CAD build for the part. Positions are in the model's coordinates, mm. Face numbers are marked on the shaded views. A direction names the side the tool comes from. Round coordinates to 2 decimals unless told otherwise and drop trailing zeros. Loops run counter-clockwise (first coordinate to the right, second up) from the corner with the lowest first, then second, coordinate; pieces in that order, holes last. Notation, with made-up numbers: M 19.25,4.5 L 49.25,4.5 A32 cw 49.25,41.5 Z; hole C 87,40 d1. An arc over 180 degrees is marked long. Put each result on its own line as item: value. Start each with the question number.
from build123d import *

# Parameters (mm, degrees)
SKETCH_1_W          = 20.1
SKETCH_1_H          = 6.6
EXTRUDE_1_DEPTH     = 1.6
CUT_EXTRUDE_1_REACH = 3.6
SKETCH_2_R          = 1
EXTRUDE_2_DEPTH     = 5
SKETCH_4_W          = 8.928427124
SKETCH_4_H          = 1
EXTRUDE_3_DEPTH     = 8
CUT_EXTRUDE_2_DEPTH = 5
EXTRUDE_4_DEPTH     = 3.5


with BuildPart() as part:
    # 草图1 → 凸台-拉伸1 (new body)
    with BuildSketch(Plane(origin=(0, 0, 0), x_dir=(1, 0, 0), z_dir=(0, 1, 0))):
        Rectangle(SKETCH_1_W, SKETCH_1_H)
    extrude(amount=EXTRUDE_1_DEPTH)

    # 草图2 → 切除-拉伸1 (cut, up to next)
    with BuildSketch(Plane(origin=(0, 1.6, 0), x_dir=(1, 0, 0), z_dir=(0, 1, 0)), mode=Mode.PRIVATE) as cut_extrude_1_sk1:
        with Locations((8, 0)):
            Circle(SKETCH_2_R)
    cut_extrude_1_tool1 = extrude(cut_extrude_1_sk1.sketch, amount=-CUT_EXTRUDE_1_REACH, mode=Mode.PRIVATE) & part.part
    add(cut_extrude_1_tool1.solids().sort_by_distance((8, 1.6, 0))[0], mode=Mode.SUBTRACT)
    # 草图2 → 切除-拉伸1 (cut, up to next)
    with BuildSketch(Plane(origin=(0, 1.6, 0), x_dir=(1, 0, 0), z_dir=(0, 1, 0)), mode=Mode.PRIVATE) as cut_extrude_1_sk2:
        with Locations((-8, 0)):
            Circle(SKETCH_2_R)
    cut_extrude_1_tool2 = extrude(cut_extrude_1_sk2.sketch, amount=-CUT_EXTRUDE_1_REACH, mode=Mode.PRIVATE) & part.part
    add(cut_extrude_1_tool2.solids().sort_by_distance((-8, 1.6, 0))[0], mode=Mode.SUBTRACT)

    # 草图3 → 凸台-拉伸2 (add)
    with BuildSketch(Plane.XZ):
        with BuildLine():
            Line((-3.05, 1.5), (3.05, 1.5))
            ThreePointArc((3.05, 1.5), (4.55, 0), (3.05, -1.5))
            Line((3.05, -1.5), (-3.05, -1.5))
            ThreePointArc((-3.05, -1.5), (-4.55, 0), (-3.05, 1.5))
        make_face()
    extrude(amount=EXTRUDE_2_DEPTH)

    # 草图4 → 凸台-拉伸3 (add)
    with BuildSketch(Plane.XZ.offset(5)):
        Rectangle(SKETCH_4_W, SKETCH_4_H)
    extrude(amount=EXTRUDE_3_DEPTH)

    # 草图5 → 切除-拉伸2 (cut)
    with BuildSketch(Plane(origin=(0, 1.6, 0), x_dir=(1, 0, 0), z_dir=(0, 1, 0))):
        with BuildLine():
            Line((-2.95, 1.3), (2.95, 1.3))
            ThreePointArc((2.95, 1.3), (4.25, 0), (2.95, -1.3))
            Line((2.95, -1.3), (-2.95, -1.3))
            ThreePointArc((-2.95, -1.3), (-4.25, 0), (-2.95, 1.3))
        make_face()
    extrude(amount=-CUT_EXTRUDE_2_DEPTH, mode=Mode.SUBTRACT)

    # 草图6 → 凸台-拉伸4 (add)
    with BuildSketch(Plane(origin=(0, -3.4, 0), x_dir=(1, 0, 0), z_dir=(0, 1, 0))):
        with BuildLine():
            Line((-3.05, -0.4), (3.05, -0.4))
            ThreePointArc((3.05, -0.4), (3.191421356, -0.341421356), (3.25, -0.2))
            Line((3.25, -0.2), (3.25, 0.2))
            ThreePointArc((3.25, 0.2), (3.191421356, 0.341421356), (3.05, 0.4))
            Line((3.05, 0.4), (-3.05, 0.4))
            ThreePointArc((-3.05, 0.4), (-3.191421356, 0.341421356), (-3.25, 0.2))
            Line((-3.25, 0.2), (-3.25, -0.2))
            ThreePointArc((-3.25, -0.2), (-3.191421356, -0.341421356), (-3.05, -0.4))
        make_face()
    extrude(amount=EXTRUDE_4_DEPTH)


solid = part.part
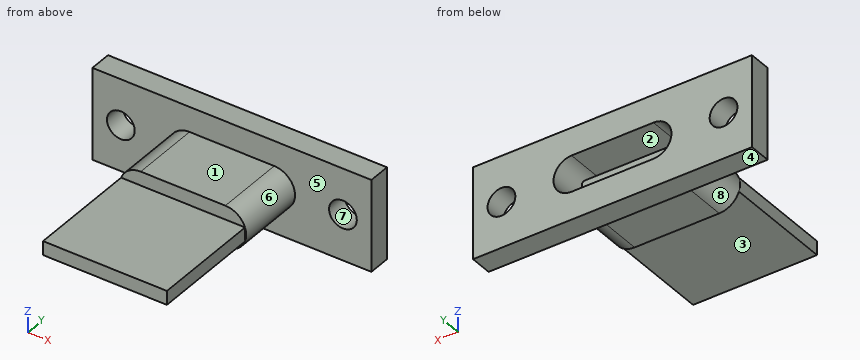
(1) Cut at D-D on y = -4.25. List the corners of the cut face in (x, z).
(2) Drill centre lines: line 1 along X through (y, z) = (1.05, 0); line 2 along Z through (x, y) = (1.75, -3.25); line 3 along Z through (x, y) = (-8, 0.85). Where is each one in solid material? Low to high.
(3) Tool access for the marked faces 1, 2, 3 and 4: list every direction of +Z, -Z, +X, -X, +Y, -Y with a clear straight run to the whole face (end or side of a thin tool).
(4) Cut at C-C on x = -0.5. List the corners of the cut face in (y, z), and give its area (3 significant figures).
(5) Cut at A-A on y = -1.5. List the corners of the cut face in (x, z), and give its area (3 significant figures).
(6) Flat gauge pins, fed straight in: pin 1 Ø1.8 at (x, y) = (1, -1.5) entering from +Z; pin 2 Ø1.8 at (x, z) = (8, 0) entering from +Y; pin 3 Ø5 at (x, y) = (-6.5, -3.5) entering from -Z; pin 4 Ø0.5 at (x, z) = (-1.5, -1) entering from -Y. Where does each tip first touch, or does it go through?
(7) Mould opens along X. For the marked faces 5, 6, 7 and 8 say: +X half, -X half, draft (parallel to the pull), parting line (faces both ways), or undercut.
(8) Cut at B-B on x = -8. List the corners of the cut face in (y, z), and give its area (3 significant figures).
Taken from the geometry:
1. outline: M -3.05,-1.5 L 3.05,-1.5 A1.5 ccw 3.05,1.5 L -3.05,1.5 A1.5 ccw Z
2. line 1: -10.05 to -9, -7 to -4.25, 4.25 to 7, 9 to 10.05
2. line 2: -1.5 to -1.3, -0.4 to 0.4, 1.3 to 1.5
2. line 3: -3.3 to -1, 1 to 3.3
3. face 1: +Z, +X, -X, -Y
3. face 2: +Y
3. face 3: -Z, +X, -X, -Y
3. face 4: -Z, +X, -X, +Y, -Y
4. outline: M -13,-0.5 L -5,-0.5 L -5,-1.5 L 0,-1.5 L 0,-3.3 L 1.6,-3.3 L 1.6,-1.3 L -3.4,-1.3 L -3.4,-0.4 L 0.1,-0.4 L 0.1,0.4 L -3.4,0.4 L -3.4,1.3 L 1.6,1.3 L 1.6,3.3 L 0,3.3 L 0,1.5 L -5,1.5 L -5,0.5 L -13,0.5 Z
4. area: 23.4 mm2
5. outline: M -3.25,-0.2 A0.2 ccw -3.05,-0.4 L 3.05,-0.4 A0.2 ccw 3.25,-0.2 L 3.25,0.2 A0.2 ccw 3.05,0.4 L -3.05,0.4 A0.2 ccw -3.25,0.2 Z; M -3.05,-1.5 L 3.05,-1.5 A1.5 ccw 3.05,1.5 L -3.05,1.5 A1.5 ccw Z; hole M -2.95,-1.3 L 2.95,-1.3 A1.3 ccw 2.95,1.3 L -2.95,1.3 A1.3 ccw Z
5. area: 9.88 mm2
6. pin 1: z = 1.5
6. pin 2: through
6. pin 3: z = -1.16
6. pin 4: y = -5
7. face 5: draft
7. face 6: +X half
7. face 7: undercut
7. face 8: -X half
8. outline: M 0,-3.3 L 1.6,-3.3 L 1.6,-1 L 0,-1 Z; M 0,1 L 1.6,1 L 1.6,3.3 L 0,3.3 Z
8. area: 7.36 mm2
